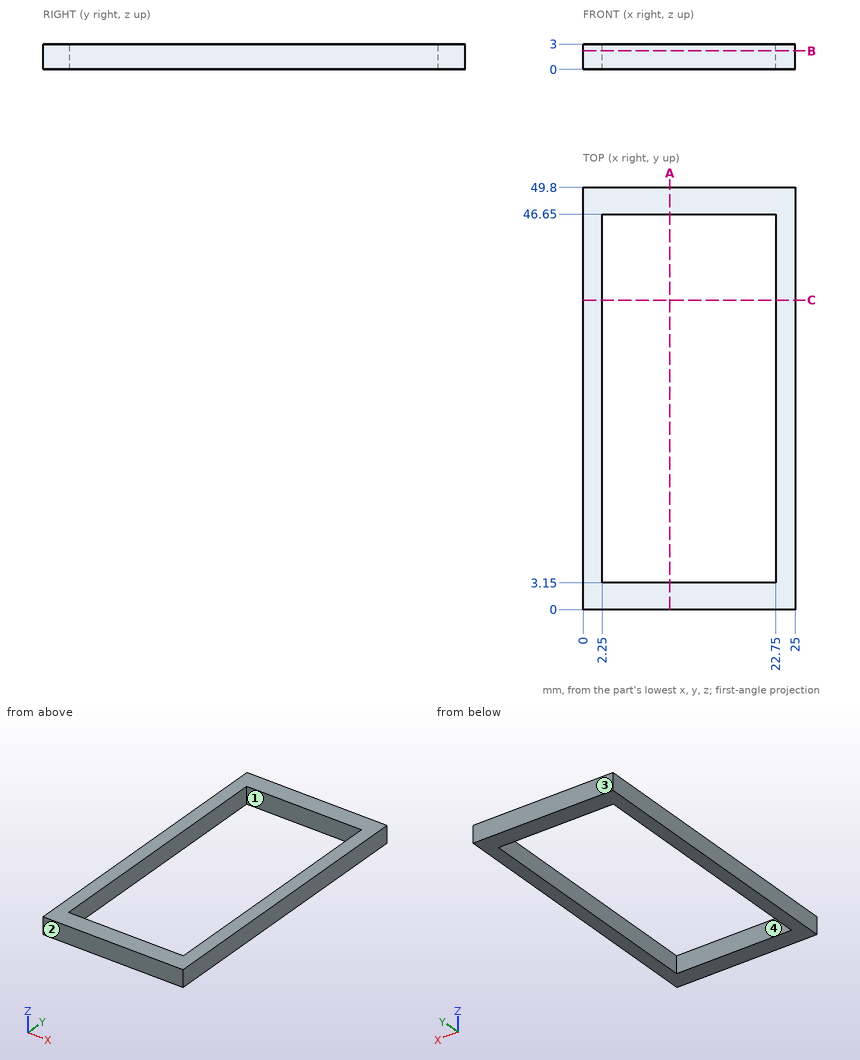
Here's the drawing with two shaded views (mm, measured from the low corner). I have some questions. A direction names the side the tool comes from. Coordinates: 2 decimals unless noted, no trailing zeros. Write each loop counter-clockwise with the first axis right and the second up, starting at its lowest first coordinate (ties: lowest second). Pieces come first, ordered by that corner, then holes. Notation, with made-up numbers: (7, 28) - (41, 28) arc R31 cw to (41, 53) - close; hole circle Ø1 at (36.5, 44). An arc over 180 degrees is marked (long way). Return JSON: item names as keys, results as strings.
Q1. Please list where these lines run through material, in increasing order: L1, parallel to X at y = 28, z = 2.65; L2, parallel to Y at x = 10, z = 2.6. Write a range as from..to.
Computed values:
{"L1": "x = 0..2.25, 22.75..25", "L2": "y = 0..3.15, 46.65..49.8"}
Q2. On a 3-axis mill with a long thin cutter (end or side, diameter ignored), from which of +Z, -Z, +X, -X, +Y, -Y can I reach the whole of each face in a straight line? I mean the marked faces 1 and 2. Say none if no direction works.
Computed values:
{"face 1": "+Z, -Z", "face 2": "+Z, -Z, +X, -X, -Y"}
Q3. Thinking about a two-plate mould opening in X: for the marked faces 3 and 4, which applies, +X half, -X half, draft (parallel to the pull), parting line (faces both ways), or undercut?
Computed values:
{"face 3": "draft", "face 4": "undercut"}
Q4. If we section it at B-B (z = 2.2): Please give me the cut outline in (x, y), then the cut area to 3 significant figures.
Computed values:
{"outline": "(0, 0) - (25, 0) - (25, 49.8) - (0, 49.8) - close; hole (2.25, 3.15) - (22.75, 3.15) - (22.75, 46.65) - (2.25, 46.65) - close", "area": "353 mm2"}
Q5. If we section it at A-A (x = 10.25): Please give me the cut outline in (y, z), then the cut area to 3 significant figures.
Computed values:
{"outline": "(0, 0) - (3.15, 0) - (3.15, 3) - (0, 3) - close; (46.65, 0) - (49.8, 0) - (49.8, 3) - (46.65, 3) - close", "area": "18.9 mm2"}
Q6. If we section it at C-C (y = 36.5): Please give me the cut outline in (x, z), then the cut area to 3 significant figures.
Computed values:
{"outline": "(0, 0) - (2.25, 0) - (2.25, 3) - (0, 3) - close; (22.75, 0) - (25, 0) - (25, 3) - (22.75, 3) - close", "area": "13.5 mm2"}
Q7. I'm going to push a flat-ended pin straight in: pin 1 Ø6 at (x, y) = (10.5, 43) entering from -Z. Where does the tip first touch, or does it pass through?
Computed values:
{"pin 1": "passes through"}
